The model under review builds one solid part; all positions refer to its coordinate system, in mm. A direction names the side the tool comes from. Round coordinates to 2 decimals unless told otherwise and drop trailing zeros. Order: outer loops, then holes, each group sorted by start corner. A loop starts at its lowest first (then second) coordinate and runs counter-clockwise, first axis right, second up. Notation, with made-up numbers: M 10.25,58.25 L 17.25,58.25 A36 ccw 17.25,94.25 Z; hole C 23,-29.5 d2. An arc over 180 degrees is marked long. Answer as a JSON object with one key per item and string values. Group by question number.
1) Consider section C-C, the plane y = -12.25. Write out the cut boundary in (x, z).
2) Insertion check: pin 1 Ø15 at (y, z) = (-17.5, 47.5) entering from -X; pin 2 Ø2.5 at (x, z) = (34, 80) entering from -Y (1 decimal). Each pin has a flat end and moves straight along its axis. Give the tip position at first contact, or say it passes through.
3) For faces 5 (the cylindrical face through (6.09, -52.54, 77.9)), 6 (the flat face through (97, -25, 44)), list the 3-axis set-ups (+Z, -Z, +X, -X, +Y, -Y) from which the entire face can be reached by the end or side of a thin tool; tool diameter is ignored.
4) Consider section A-A, the plane x = 6. Write out the cut boundary in (y, z).
5) Consider section B-B, the plane z = 80. Write out the cut boundary in (x, y).
6) To check wall thickness, follow line 1 (Z direction, x = 6, y = -51.25); line 2 (X direction, y = -53.7, z = 40); line 3 (Y direction, x = 86, z = 45). State the ranges of each line that lie inside material, in increasing order.
7) The part is to be moulded in two halves that separate along Z. For faces 1 (the flat face through (59, -52, 90)), 2 (the cylindrical face through (6.09, 2.47, 77.9)), 3 (the flat face through (0, -53, 44)), 4 (the cylindrical face through (31.95, -52.54, 39.54)), say which applies: +Z half, -Z half, draft (parallel to the pull), parting line (faces both ways), or undercut.
8) Consider section D-D, the plane z = 67. Write out the cut boundary in (x, y).
```python
from build123d import *

# Parameters (mm, degrees)
EXTRUDE_1_DEPTH         = 90
CUT_EXTRUDE1_DEPTH      = 147.727638841
CUT_EXTRUDE1_DEPTH_BACK = 147.727638841
SKETCH1_R               = 2.1
SKETCH_2_R              = 4.25
CUT_EXTRUDE_1_DEPTH     = 144.296894593


with BuildPart() as part:
    # 草图1 → 凸台-拉伸1 (new body)
    with BuildSketch(Plane.XY):
        Polygon((0, 0), (0, 5), (102, 5), (102, -55), (0, -55), (0, -50), (97, -50), (97, 0), align=None)
    extrude(amount=EXTRUDE_1_DEPTH)

    # Sketch1 → Cut-Extrude1 (cut, two sides: drawn at the far end of the back side and taken through both)
    with BuildSketch(Plane(origin=(0, 0, 0), x_dir=(1, 0, 0), z_dir=(0, 1, 0)).offset(-CUT_EXTRUDE1_DEPTH_BACK)):
        with Locations(Location((6, -40, 0), (0, 0, 270))):
            Circle(SKETCH1_R)
        with Locations(Location((34, -40, 0), (0, 0, 270))):
            Circle(SKETCH1_R)
        with Locations(Location((34, -80, 0), (0, 0, 270))):
            Circle(SKETCH1_R)
        with Locations(Location((6, -80, 0), (0, 0, 270))):
            Circle(SKETCH1_R)
    extrude(amount=CUT_EXTRUDE1_DEPTH + CUT_EXTRUDE1_DEPTH_BACK, mode=Mode.SUBTRACT)

    # 草图2 → 切除-拉伸1 (cut, through all)
    with BuildSketch(Plane.ZY.offset(-97)):
        with Locations((13, -12.25)):
            Circle(SKETCH_2_R)
    extrude(amount=-CUT_EXTRUDE_1_DEPTH, mode=Mode.SUBTRACT)


solid = part.part
```
Results list:
{
 "1": {"outline": "M 97,0 L 102,0 L 102,8.75 L 97,8.75 Z; M 97,17.25 L 102,17.25 L 102,90 L 97,90 Z"},
 "2": {"pin 1": "x = 97", "pin 2": "through"},
 "3": {"face 5": "+Y, -Y", "face 6": "+Z, -Z, -X"},
 "4": {"outline": "M -55,0 L -50,0 L -50,37.9 L -55,37.9 Z; M -55,42.1 L -50,42.1 L -50,77.9 L -55,77.9 Z; M -55,82.1 L -50,82.1 L -50,90 L -55,90 Z; M 0,0 L 5,0 L 5,37.9 L 0,37.9 Z; M 0,42.1 L 5,42.1 L 5,77.9 L 0,77.9 Z; M 0,82.1 L 5,82.1 L 5,90 L 0,90 Z"},
 "5": {"outline": "M 0,-55 L 3.9,-55 L 3.9,-50 L 0,-50 Z; M 0,0 L 3.9,0 L 3.9,5 L 0,5 Z; M 8.1,-55 L 31.9,-55 L 31.9,-50 L 8.1,-50 Z; M 8.1,0 L 31.9,0 L 31.9,5 L 8.1,5 Z; M 36.1,-55 L 102,-55 L 102,5 L 36.1,5 L 36.1,0 L 97,0 L 97,-50 L 36.1,-50 Z"},
 "6": {"line 1": "0 to 37.9, 42.1 to 77.9, 82.1 to 90", "line 2": "0 to 3.9, 8.1 to 31.9, 36.1 to 102", "line 3": "-55 to -50, 0 to 5"},
 "7": {"face 1": "+Z half", "face 2": "undercut", "face 3": "draft", "face 4": "undercut"},
 "8": {"outline": "M 0,-55 L 102,-55 L 102,5 L 0,5 L 0,0 L 97,0 L 97,-50 L 0,-50 Z"}
}
